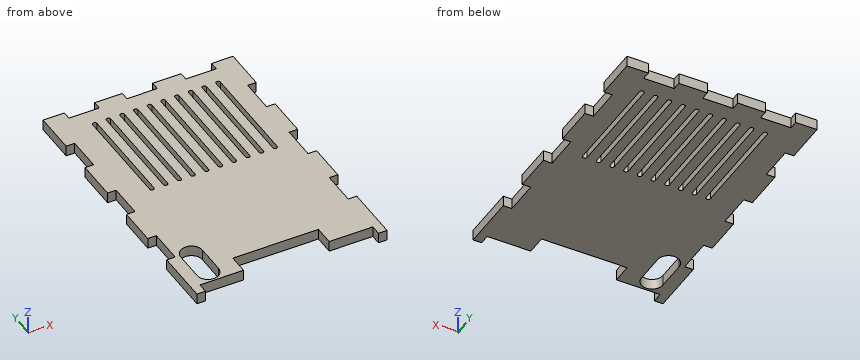
from build123d import *

# Parameters (mm, degrees)
RESSALTO_EXTRUS_O1_DEPTH = 2.5


with BuildPart() as part:
    # Esboço1 → Ressalto-extrusão1 (new body)
    with BuildSketch(Plane.XY):
        Polygon((-25.098396903, -50.388461043), (-23.098396903, -50.388461043), (-23.098396903, -47.988461043), (-12.898396903, -47.988461043), (-12.898396903, -43.388461043), (7.101603097, -43.388461043), (7.101603097, -47.988461043), (17.301603097, -47.988461043), (17.301603097, -50.388461043), (19.301603097, -50.388461043), (19.301603097, -37.412155135), (17.301603097, -37.412155135), (17.301603097, -29.312155135), (19.301603097, -29.312155135), (19.301603097, -20.19154649), (17.301603097, -20.19154649), (17.301603097, -12.09154649), (19.301603097, -12.09154649), (19.301603097, -2.411827174), (17.301603097, -2.411827174), (17.301603097, 5.688172826), (19.301603097, 5.688172826), (19.301603097, 15.611538957), (14.281603097, 15.611538957), (14.281603097, 13.615257293), (7.181603097, 13.615257293), (7.181603097, 15.611538957), (0.521603097, 15.611538957), (0.521603097, 13.615257293), (-6.578396903, 13.615257293), (-6.578396903, 15.611538957), (-13.018396903, 15.611538957), (-13.018396903, 13.615257293), (-20.118396903, 13.615257293), (-20.118396903, 15.611538957), (-25.098396903, 15.611538957), (-25.098396903, 5.691538957), (-23.098396903, 5.691538957), (-23.098396903, -2.408461043), (-25.098396903, -2.408461043), (-25.098396903, -12.088461043), (-23.098396903, -12.088461043), (-23.098396903, -20.188461043), (-25.098396903, -20.188461043), (-25.098396903, -29.308461043), (-23.098396903, -29.308461043), (-23.098396903, -37.408461043), (-25.098396903, -37.408461043), align=None)
        with BuildLine():
            ThreePointArc((-22.098396903, -37.988461043), (-19.598396903, -35.488461043), (-17.098396903, -37.988461043))
            Line((-17.098396903, -37.988461043), (-17.098396903, -44.988461043))
            ThreePointArc((-17.098396903, -44.988461043), (-19.598396903, -47.488461043), (-22.098396903, -44.988461043))
            Line((-22.098396903, -44.988461043), (-22.098396903, -37.988461043))
        make_face(mode=Mode.SUBTRACT)
        with BuildLine():
            ThreePointArc((-16.898396903, 9.334849068), (-16.398396903, 9.834849068), (-15.898396903, 9.334849068))
            Line((-15.898396903, 9.334849068), (-15.898396903, -15.047771388))
            ThreePointArc((-15.898396903, -15.047771388), (-16.398396903, -15.547771388), (-16.898396903, -15.047771388))
            Line((-16.898396903, -15.047771388), (-16.898396903, 9.334849068))
        make_face(mode=Mode.SUBTRACT)
        with BuildLine():
            ThreePointArc((-13.698396903, 9.334849068), (-13.198396903, 9.834849068), (-12.698396903, 9.334849068))
            Line((-12.698396903, 9.334849068), (-12.698396903, -15.047771388))
            ThreePointArc((-12.698396903, -15.047771388), (-13.198396903, -15.547771388), (-13.698396903, -15.047771388))
            Line((-13.698396903, -15.047771388), (-13.698396903, 9.334849068))
        make_face(mode=Mode.SUBTRACT)
        with BuildLine():
            ThreePointArc((-10.498396903, 9.334849068), (-9.998396903, 9.834849068), (-9.498396903, 9.334849068))
            Line((-9.498396903, 9.334849068), (-9.498396903, -15.047771388))
            ThreePointArc((-9.498396903, -15.047771388), (-9.998396903, -15.547771388), (-10.498396903, -15.047771388))
            Line((-10.498396903, -15.047771388), (-10.498396903, 9.334849068))
        make_face(mode=Mode.SUBTRACT)
        with BuildLine():
            ThreePointArc((-7.298396903, 9.334849068), (-6.798396903, 9.834849068), (-6.298396903, 9.334849068))
            Line((-6.298396903, 9.334849068), (-6.298396903, -15.047771388))
            ThreePointArc((-6.298396903, -15.047771388), (-6.798396903, -15.547771388), (-7.298396903, -15.047771388))
            Line((-7.298396903, -15.047771388), (-7.298396903, 9.334849068))
        make_face(mode=Mode.SUBTRACT)
        with BuildLine():
            ThreePointArc((-4.098396903, 9.334849068), (-3.598396903, 9.834849068), (-3.098396903, 9.334849068))
            Line((-3.098396903, 9.334849068), (-3.098396903, -15.047771388))
            ThreePointArc((-3.098396903, -15.047771388), (-3.598396903, -15.547771388), (-4.098396903, -15.047771388))
            Line((-4.098396903, -15.047771388), (-4.098396903, 9.334849068))
        make_face(mode=Mode.SUBTRACT)
        with BuildLine():
            ThreePointArc((-0.898396903, 9.334849068), (-0.398396903, 9.834849068), (0.101603097, 9.334849068))
            Line((0.101603097, 9.334849068), (0.101603097, -15.047771388))
            ThreePointArc((0.101603097, -15.047771388), (-0.398396903, -15.547771388), (-0.898396903, -15.047771388))
            Line((-0.898396903, -15.047771388), (-0.898396903, 9.334849068))
        make_face(mode=Mode.SUBTRACT)
        with BuildLine():
            ThreePointArc((2.301603097, 9.334849068), (2.801603097, 9.834849068), (3.301603097, 9.334849068))
            Line((3.301603097, 9.334849068), (3.301603097, -15.047771388))
            ThreePointArc((3.301603097, -15.047771388), (2.801603097, -15.547771388), (2.301603097, -15.047771388))
            Line((2.301603097, -15.047771388), (2.301603097, 9.334849068))
        make_face(mode=Mode.SUBTRACT)
        with BuildLine():
            ThreePointArc((5.501603097, 9.334849068), (6.001603097, 9.834849068), (6.501603097, 9.334849068))
            Line((6.501603097, 9.334849068), (6.501603097, -15.047771388))
            ThreePointArc((6.501603097, -15.047771388), (6.001603097, -15.547771388), (5.501603097, -15.047771388))
            Line((5.501603097, -15.047771388), (5.501603097, 9.334849068))
        make_face(mode=Mode.SUBTRACT)
        with BuildLine():
            ThreePointArc((8.701603097, 9.334849068), (9.201603097, 9.834849068), (9.701603097, 9.334849068))
            Line((9.701603097, 9.334849068), (9.701603097, -15.047771388))
            ThreePointArc((9.701603097, -15.047771388), (9.201603097, -15.547771388), (8.701603097, -15.047771388))
            Line((8.701603097, -15.047771388), (8.701603097, 9.334849068))
        make_face(mode=Mode.SUBTRACT)
        with BuildLine():
            ThreePointArc((11.901603097, 9.334849068), (12.401603097, 9.834849068), (12.901603097, 9.334849068))
            Line((12.901603097, 9.334849068), (12.901603097, -15.047771388))
            ThreePointArc((12.901603097, -15.047771388), (12.401603097, -15.547771388), (11.901603097, -15.047771388))
            Line((11.901603097, -15.047771388), (11.901603097, 9.334849068))
        make_face(mode=Mode.SUBTRACT)
    extrude(amount=RESSALTO_EXTRUS_O1_DEPTH)


solid = part.part
Input: part model. Units: mm. Frame: model coordinates. Coordinates: 2 decimals unless noted, no trailing zeros. Loops run counter-clockwise (first coordinate to the right, second up) from the corner with the lowest first, then second, coordinate; pieces in that order, holes last. Notation, with made-up numbers: (47.5, -23.75) -> (103.5, -23.75) arc R18 ccw to (103.5, -13.75) -> close; hole circle Ø4 at (-2.5, 7). An arc over 180 degrees is marked (long way). Write each question's results on one line, items separated by ' | '. Start each with the question number.
Q1. Ray query, line 1 (X direction, y = -38.5, z = 2); line 2 (Y direction, x = -16.5, z = 2.3); line 3 (Y direction, x = 8.5, z = 1.35). Return the intervals inside material, ascending. Write a range as from..to.
Q2. Section A-A, the plane x = -21. Return the cut outline in (y, z).
Q3. Section B-B, the plane z = 1.95. State how many separate pieces and enclosed holes the cut face has, plus the area to 3 significant figures.
Q4. Pin query (flat end, axial travel): pin 1 (1.2 mm diameter, centred on y = 2.5, z = 0.5, fed in from +X); pin 2 (1.5 mm diameter, centred on y = -18.5, z = 1, fed in from -X). Return the tip coordinate at first contact, or that it passes through.
Found:
1) line 1: -25.1..-22.1, -17.1..19.3 | line 2: -47.99..-15.54, 9.82..13.62 | line 3: -47.99..13.62
2) outline: (-47.99, 0) -> (-47.06, 0) -> (-47.06, 2.5) -> (-47.99, 2.5) -> close; (-35.92, 0) -> (15.61, 0) -> (15.61, 2.5) -> (-35.92, 2.5) -> close
3) separate pieces: 1 | enclosed holes: 11 | area: 2,300 mm2
4) pin 1: x = 17.3 | pin 2: x = -23.1
